from build123d import *

# Parameters (mm, degrees)
CYLINDER001_R           = 1.8
CYLINDER001_DEPTH       = 3.23
THICKNESS002_T          = -1.1
CYLINDER003_R           = 1.8
CYLINDER003_DEPTH       = 3.23
THICKNESS003_T          = -1.1
CYLINDER006_R           = 0.7
CYLINDER006_DEPTH       = 3
CYLINDER006_ROLL_ANGLE  = -90
CYLINDER005_R           = 0.7
CYLINDER005_DEPTH       = 3
CYLINDER005_PITCH_ANGLE = 90
CYLINDER004_R           = 0.7
CYLINDER004_DEPTH       = 10
CYLINDER002_R           = 0.7
CYLINDER002_DEPTH       = 10
BOX001_W                = 8.6
BOX001_H                = 8.6
BOX001_DEPTH            = 1.77
CYLINDER_R              = 14
CYLINDER_DEPTH          = 8
THICKNESS_T             = 1.77
BOX_W                   = 15.9
BOX_H                   = 15.9
BOX_DEPTH               = 3.23
THICKNESS001_T          = -1.771


with BuildPart() as thickness002:
    # Cylinder001 → Cylinder001 (new body)
    with BuildSketch(Plane.XY):
        Circle(CYLINDER001_R)
    extrude(amount=CYLINDER001_DEPTH)

    # Thickness002
    thickness002_openings = [thickness002.faces().sort_by_distance(p)[0] for p in [
        (0, 0, 3.23),
        (0, 0, 0),
    ]]
    offset(amount=THICKNESS002_T, openings=thickness002_openings)


with BuildPart() as thickness002_1:
    # Thickness002 placement: moved
    add(thickness002.part.moved(Location((9.75, 0, 0))))


with BuildPart() as thickness003:
    # Cylinder003 → Cylinder003 (new body)
    with BuildSketch(Plane.XY):
        Circle(CYLINDER003_R)
    extrude(amount=CYLINDER003_DEPTH)

    # Thickness003
    thickness003_openings = [thickness003.faces().sort_by_distance(p)[0] for p in [
        (0, 0, 3.23),
        (0, 0, 0),
    ]]
    offset(amount=THICKNESS003_T, openings=thickness003_openings)


with BuildPart() as thickness003_1:
    # Thickness003 placement: moved
    add(thickness003.part.moved(Location((-9.75, 0, 0))))


with BuildPart() as cylinder006:
    # Cylinder006 → Cylinder006 (new body)
    with BuildSketch(Plane.XY):
        Circle(CYLINDER006_R)
    extrude(amount=CYLINDER006_DEPTH)


with BuildPart() as cylinder006_1:
    # Cylinder006 roll: moved
    add(cylinder006.part.rotate(Axis((0, 0, 0), (1, 0, 0)), CYLINDER006_ROLL_ANGLE))


with BuildPart() as cylinder006_2:
    # Cylinder006 placement: moved
    add(cylinder006_1.part.moved(Location((0, 13, 10.7))))


with BuildPart() as cylinder005:
    # Cylinder005 → Cylinder005 (new body)
    with BuildSketch(Plane.XY):
        Circle(CYLINDER005_R)
    extrude(amount=CYLINDER005_DEPTH)


with BuildPart() as cylinder005_1:
    # Cylinder005 pitch: moved
    add(cylinder005.part.rotate(Axis((0, 0, 0), (0, 1, 0)), CYLINDER005_PITCH_ANGLE))


with BuildPart() as cylinder005_2:
    # Cylinder005 placement: moved
    add(cylinder005_1.part.moved(Location((13, 0, 10.7))))


with BuildPart() as cylinder004:
    # Cylinder004 → Cylinder004 (new body)
    with BuildSketch(Plane(origin=(-9.75, 0, 0), x_dir=(1, 0, 0), z_dir=(0, 0, 1))):
        Circle(CYLINDER004_R)
    extrude(amount=CYLINDER004_DEPTH)


with BuildPart() as cylinder002:
    # Cylinder002 → Cylinder002 (new body)
    with BuildSketch(Plane(origin=(9.75, 0, 0), x_dir=(1, 0, 0), z_dir=(0, 0, 1))):
        Circle(CYLINDER002_R)
    extrude(amount=CYLINDER002_DEPTH)


with BuildPart() as cube001:
    # Box001 → Box001 (new body)
    with BuildSketch(Plane(origin=(-4.3, -4.3, 3.23), x_dir=(1, 0, 0), z_dir=(0, 0, 1))):
        with Locations((4.3, 4.3)):
            Rectangle(BOX001_W, BOX001_H)
    extrude(amount=BOX001_DEPTH)


with BuildPart() as cut004:
    # Cylinder → Cylinder (new body)
    with BuildSketch(Plane.XY.offset(5)):
        Circle(CYLINDER_R)
    extrude(amount=CYLINDER_DEPTH)

    # Thickness
    thickness_openings = [cut004.faces().sort_by_distance(p)[0] for p in [
        (0, 0, 13),
    ]]
    offset(amount=THICKNESS_T, openings=thickness_openings, kind=Kind.INTERSECTION)

    # Cut: cut Cube001
    add(cube001.part, mode=Mode.SUBTRACT)

    # Cut001: cut Cylinder002
    add(cylinder002.part, mode=Mode.SUBTRACT)

    # Cut002: cut Cylinder004
    add(cylinder004.part, mode=Mode.SUBTRACT)

    # Cut003: cut Cylinder005
    add(cylinder005_2.part, mode=Mode.SUBTRACT)

    # Cut004: cut Cylinder006
    add(cylinder006_2.part, mode=Mode.SUBTRACT)


with BuildPart() as fusion:
    # Box → Box (new body)
    with BuildSketch(Plane(origin=(-7.95, -7.95, 0), x_dir=(1, 0, 0), z_dir=(0, 0, 1))):
        with Locations((7.95, 7.95)):
            Rectangle(BOX_W, BOX_H)
    extrude(amount=BOX_DEPTH)

    # Thickness001
    thickness001_openings = [fusion.faces().sort_by_distance(p)[0] for p in [
        (0, 0, 3.23),
        (0, 0, 0),
    ]]
    offset(amount=THICKNESS001_T, openings=thickness001_openings, kind=Kind.INTERSECTION)

    # Fusion: union Thickness002, Thickness003, Cut004
    add(thickness002_1.part)
    add(thickness003_1.part)
    add(cut004.part)


solid = fusion.part
Work out the finished part from the listing and answer in its coordinate system (mm). A direction names the side the tool comes from. Give positions to 0.01 mm unless a question says otherwise; leave off trailing zeros. Write each loop counter-clockwise with the first axis right and the second up, starting at its lowest first coordinate (ties: lowest second). Pieces come first, ordered by that corner, then holes. Notation, with made-up numbers: (46.5, 49) - (91.5, 49) arc R30 ccw to (91.5, 82) - close; hole circle Ø4 at (-11, 6). An arc over 180 degrees is marked (long way). One line per item, written item: value. Start each with the question number.
1. Find section B-B (x = 0). Write down the section's boundary in (y, z).
2. Consider probe 1 along Y at (x, z) = (9.75, 1.85); probe 2 along Y at (x, z) = (-2.5, 1.75). Determine where each line is inside the solid, lowest interval first.
3. For a pull along X with two mould halves and no side action, classify faces 1 (the flat face through (7, 0, 0)), 2 (the cylindrical face through (-11.62, 10.66, 8.05)), 3 (the flat face through (7.95, -4, 2)) as +X half, -X half, draft (parallel to the pull), parting line (faces both ways), or undercut.
4. For faces 4 (the flat face through (-4.3, 0, 4)), 5 (the flat face through (6.179, 0, 2)), 6 (the flat face through (6, 0, 5)), 7 (the flat face through (0, 7.95, 2)), determine the directions among +Z, -Z, +X, -X, +Y, -Y from which every point of the face is accessible in a straight line to the end or side of a thin tool.
5. Given pin 1 (3.5 mm diameter, centred on x = 2.5, z = 2, fed in from -Y); pin 2 (13.5 mm diameter, centred on x = -1, y = -1, fed in from -Z); pin 3 (1.6 mm diameter, centred on y = -2.5, z = 2.5, fed in from -X); pin 4 (3 mm diameter, centred on x = -11.5, z = 3, fed in from +Y), each flat-ended and moving along its own axis, determine where each tip first touches the part or whether it passes through.
6. Find section D-D (z = 8.5). Write down the section's boundary in (x, y), then the cut area to 3 significant figures.
7. Find section C-C (x = -9.75). Write down the section's boundary in (y, z).
Geometry results:
1. outline: (-15.77, 3.23) - (-7.95, 3.23) - (-7.95, 0) - (-6.18, 0) - (-6.18, 3.23) - (-4.3, 3.23) - (-4.3, 5) - (-14, 5) - (-14, 13) - (-15.77, 13) - close; (4.3, 3.23) - (6.18, 3.23) - (6.18, 0) - (7.95, 0) - (7.95, 3.23) - (15.77, 3.23) - (15.77, 10) - (14, 10) - (14, 5) - (4.3, 5) - close; (14, 11.4) - (15.77, 11.4) - (15.77, 13) - (14, 13) - close
2. probe 1: -1.8 to -0.7, 0.7 to 1.8
2. probe 2: -7.95 to -6.18, 6.18 to 7.95
3. face 1: draft
3. face 2: parting line
3. face 3: undercut
4. face 4: +Z, -Z
4. face 5: -Z
4. face 6: +Z
4. face 7: -Z, +X, -X, +Y
5. pin 1: y = -15.72
5. pin 2: z = 0
5. pin 3: x = -15.62
5. pin 4: y = 12.18
6. outline: circle Ø31.54 at (0, 0); hole circle Ø28 at (0, 0)
6. area: 166 mm2
7. outline: (-12.39, 3.23) - (-1.8, 3.23) - (-1.8, 0) - (-0.7, 0) - (-0.7, 5) - (-10.05, 5) - (-10.05, 13) - (-12.39, 13) - close; (0.7, 0) - (1.8, 0) - (1.8, 3.23) - (12.39, 3.23) - (12.39, 13) - (10.05, 13) - (10.05, 5) - (0.7, 5) - close
